```python
from build123d import *

# Parameters (mm, degrees)
F0_W     = 152.4
F0_H     = 152.4
F1_DEPTH = 9.525
F3_D     = 3.4544
F5_D     = 13.49248


with BuildPart() as f1:
    # F0 (on Top) → F1 (new body)
    with BuildSketch(Plane.XY):
        Rectangle(F0_W, F0_H)
    extrude(amount=F1_DEPTH)

    # F3 (through all)
    with Locations(Plane.XY.offset(9.525)):
        with Locations((-32.0675, -1.016), (-32.0675, -55.753), (32.0675, -55.753), (32.0675, -1.016)):
            Hole(F3_D / 2)

    # F5 (through all)
    with Locations(Plane.XY.offset(9.525)):
        with Locations((0, 0)):
            Hole(F5_D / 2)


solid = f1.part
```
Can you work these out from the model? Positions are in its coordinate system, mm. Give positions to 0.01 mm unless a question says otherwise; leave off trailing zeros. Order: outer loops, then holes, each group sorted by start corner. A loop starts at its lowest first (then second) coordinate and runs counter-clockwise, first axis right, second up. Notation, with made-up numbers: M 33.5,-19 L 80.5,-19 A24 cw 80.5,18 Z; hole C 89,-1.75 d10. An arc over 180 degrees is marked long. Write item = value, one per line. Start each with the question number.
Q1. We'd pull the mould along Y, two halves only. Please class faces 1 (the flat face through (-1, -76.2, 5)), 2 (the flat face through (16, 1, 9.525)), 3 (the cylindrical face through (-30.79, -54.59, 4.7)): pulls with the +Y half, pulls with the -Y half, needs draft (parallel to the pull), parting line crosses it, or undercut.
Q2. I need wall thicknesses on probe 1 along Y at (x, z) = (0, 6.75); probe 2 along X at (y, z) = (-57, 5); probe 3 along X at (y, z) = (3.5, 7). Which ranges of each line are inside material? Lowest first, please. Write a range as [from, to].
Q3. Suppose I cut it at A-A (x = 0). Write out the boundary of the cut face in (y, z) (3 decimals).
Check result:
q1.face_1 = pulls with the -Y half
q1.face_2 = needs draft
q1.face_3 = undercut
q2.probe_1 = [-76.2, -6.75], [6.75, 76.2]
q2.probe_2 = [-76.2, -33.26], [-30.87, 30.87], [33.26, 76.2]
q2.probe_3 = [-76.2, -5.77], [5.77, 76.2]
q3.outline = M -76.2,0 L -6.746,0 L -6.746,9.525 L -76.2,9.525 Z; M 6.746,0 L 76.2,0 L 76.2,9.525 L 6.746,9.525 Z
